```python
from build123d import *

# Parameters (mm, degrees)
SKETCH1_R           = 1.25
BOSS_EXTRUDE1_DEPTH = 3


with BuildPart() as part:
    # Sketch1 → Boss-Extrude1 (new body)
    with BuildSketch(Plane(origin=(0, 0, 0), x_dir=(1, 0, 0), z_dir=(0, 1, 0))):
        with BuildLine():
            Line((-23.25, 9), (-23.25, -9))
            Line((-23.25, -9), (23.25, -9))
            Line((23.25, -9), (23.25, 9))
            Line((23.25, 9), (15, 9))
            Line((15, 9), (15, 6.75))
            ThreePointArc((15, 6.75), (12.75, 4.5), (10.5, 6.75))
            Line((10.5, 6.75), (10.5, 9))
            Line((10.5, 9), (6.5, 9))
            Line((6.5, 9), (6.5, 6.75))
            ThreePointArc((6.5, 6.75), (4.25, 4.5), (2, 6.75))
            Line((2, 6.75), (2, 9))
            Line((2, 9), (-2, 9))
            Line((-2, 9), (-2, 6.75))
            ThreePointArc((-2, 6.75), (-4.25, 4.5), (-6.5, 6.75))
            Line((-6.5, 6.75), (-6.5, 9))
            Line((-6.5, 9), (-10.5, 9))
            Line((-10.5, 9), (-10.5, 6.75))
            ThreePointArc((-10.5, 6.75), (-12.75, 4.5), (-15, 6.75))
            Line((-15, 6.75), (-15, 9))
            Line((-15, 9), (-23.25, 9))
        make_face()
        with Locations(Location((-19.5, 0, 0), (0, 0, 270))):
            Circle(SKETCH1_R, mode=Mode.SUBTRACT)
        with Locations(Location((19.5, 0, 0), (0, 0, 270))):
            Circle(SKETCH1_R, mode=Mode.SUBTRACT)
    extrude(amount=BOSS_EXTRUDE1_DEPTH)


solid = part.part
```
Build history of the part. All positions in model axes, mm. A direction names the side the tool comes from. Round coordinates to 2 decimals unless told otherwise and drop trailing zeros. Write each loop counter-clockwise with the first axis right and the second up, starting at its lowest first coordinate (ties: lowest second). Pieces come first, ordered by that corner, then holes.
1) Drill centre lines: probe 1 along X at (y, z) = (1.65, 0); probe 2 along X at (y, z) = (2.55, -7.25); probe 3 along X at (y, z) = (2.75, -1). Where is each one in solid material? Low to high.
2) 3-axis set-ups, long thin cutter, end or side, ignore diameter. For faces 4 (the flat face through (15, 1, -8)), 5 (the flat face through (9, 1, -9)): which of +Z, -Z, +X, -X, +Y, -Y reach the whole face in a straight line?
3) Band-saw the part on D-D, the plane z = -5. List the corners of the cut face in (x, y), and give its area (3 significant figures).
4) Band-saw the part on C-C, the plane x = 19.5. List the corners of the cut face in (y, z), and give its area (3 significant figures).
5) Band-saw the part on A-A, the plane z = 0. List the corners of the cut face in (x, y).
6) Band-saw the part on B-B, the plane y = 1.7. List the corners of the cut face in (x, z), and give its area (3 significant figures).
7) Pin check, flat tips, straight feed: pin 1 (1.5 mm diameter, centred on x = 19.5, z = 0, fed in from +Y); pin 2 (4 mm diameter, centred on x = -19.5, z = 0, fed in from -Y). Stop position of each tip, or through.
8) Mould opens along X. For faces 1 (the flat face through (0, 3, 0)), 2 (the flat face through (-23.25, 1, 0)), 3 (the flat face through (6.5, 1, -8)) say: +X half, -X half, draft (parallel to the pull), parting line (faces both ways), or undercut.
Ans:
1. probe 1: x = -23.25 to -20.75, -18.25 to 18.25, 20.75 to 23.25
1. probe 2: x = -23.25 to -15, -10.5 to -6.5, -2 to 2, 6.5 to 10.5, 15 to 23.25
1. probe 3: x = -23.25 to -20.25, -18.75 to 18.75, 20.25 to 23.25
2. face 4: -Z, +Y, -Y
2. face 5: -Z, +X, -X, +Y, -Y
3. outline: (-23.25, 0) - (-14.16, 0) - (-14.16, 3) - (-23.25, 3) - close; (-11.34, 0) - (-5.66, 0) - (-5.66, 3) - (-11.34, 3) - close; (-2.84, 0) - (2.84, 0) - (2.84, 3) - (-2.84, 3) - close; (5.66, 0) - (11.34, 0) - (11.34, 3) - (5.66, 3) - close; (14.16, 0) - (23.25, 0) - (23.25, 3) - (14.16, 3) - close
3. area: 106 mm2
4. outline: (0, -9) - (3, -9) - (3, -1.25) - (0, -1.25) - close; (0, 1.25) - (3, 1.25) - (3, 9) - (0, 9) - close
4. area: 46.5 mm2
5. outline: (-23.25, 0) - (-20.75, 0) - (-20.75, 3) - (-23.25, 3) - close; (-18.25, 0) - (18.25, 0) - (18.25, 3) - (-18.25, 3) - close; (20.75, 0) - (23.25, 0) - (23.25, 3) - (20.75, 3) - close
6. outline: (-23.25, -9) - (-15, -9) - (-15, -6.75) arc R2.25 cw to (-10.5, -6.75) - (-10.5, -9) - (-6.5, -9) - (-6.5, -6.75) arc R2.25 cw to (-2, -6.75) - (-2, -9) - (2, -9) - (2, -6.75) arc R2.25 cw to (6.5, -6.75) - (6.5, -9) - (10.5, -9) - (10.5, -6.75) arc R2.25 cw to (15, -6.75) - (15, -9) - (23.25, -9) - (23.25, 9) - (-23.25, 9) - close; hole circle Ø2.5 at (-19.5, 0); hole circle Ø2.5 at (19.5, 0)
6. area: 755 mm2
7. pin 1: passes through
7. pin 2: stops at y = 0
8. face 1: draft
8. face 2: -X half
8. face 3: undercut
